from build123d import *

# Parameters (mm, degrees)
F0_R     = 3.125
F1_DEPTH = 35
F2_R     = 0.5
F4_R     = 0.5


with BuildPart() as f1:
    # F0 (on Top) → F1 (new body)
    with BuildSketch(Plane.XY):
        Circle(F0_R)
    extrude(amount=F1_DEPTH)

    # F2 (on Front) → F3 (revolve, cut)
    with BuildSketch(Plane.XZ):
        with Locations((-3, 1.679414)):
            Circle(F2_R)
    revolve(axis=Axis((0, 0, 0.03065), (0, 0, 1)), mode=Mode.SUBTRACT)

    # F4 (on Front) → F5 (revolve, cut)
    with BuildSketch(Plane.XZ):
        with Locations((-3, 33.521309)):
            Circle(F4_R)
    revolve(axis=Axis((0, 0, 20.967992), (0, 0, 1)), mode=Mode.SUBTRACT)


solid = f1.part
Input: part model. Units: mm. Frame: model coordinates. Round coordinates to 2 decimals unless told otherwise and drop trailing zeros. Order: outer loops, then holes, each group sorted by start corner. A loop starts at its lowest first (then second) coordinate and runs counter-clockwise, first axis right, second up. Notation, with made-up numbers: (-4, 35.25) - (3, 35.25) arc R20 ccw to (3, 56.25) - close; hole circle Ø1 at (51, -26). An arc over 180 degrees is marked (long way). Answer as a JSON object with one key per item and string values. Group by question number.
(1) Cut plane A-A (z = 13). Return loops of the section in (x, y) (3 decimals), then the cut area to 3 significant figures.
(2) Pin query (flat end, axial travel): P1, Ø2, axis at y = 2, z = 4, coming from the -X side. Return the tip coordinate at first contact, or that it passes through.
(3) Material intervals for probe 1 along X at (y, z) = (-0.75, 11.5); probe 2 along Y at (x, z) = (-2, 26); probe 3 along X at (y, z) = (-2.5, 13.5) (3 decimals), sorted ascending. Write a range as from..to.
(4) Cut plane B-B (y = 2.75). Count the separate pieces of the cut face and the enclosed holes in it, then the cut area to 3 significant figures.
Here are the results:
{
 "1": {"outline": "circle Ø6.25 at (0, 0)", "area": "30.7 mm^2"},
 "2": {"P1": "stops at x = -2.96"},
 "3": {"probe 1": "x = -3.03..3.03", "probe 2": "y = -2.4..2.4", "probe 3": "x = -1.875..1.875"},
 "4": {"separate pieces": "3", "enclosed holes": "0", "area": "98.3 mm^2"}
}
